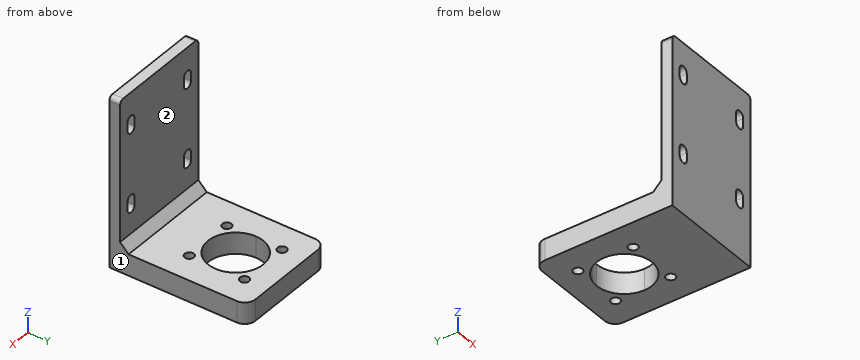
```python
from build123d import *

# Parameters (mm, degrees)
SKETCH_1_R               = 2.15
EXTRUDE_1_DEPTH          = 10
SKETCH_2_W               = 50
SKETCH_2_H               = 10
EXTRUDE_2_DEPTH          = 5
SKETCH_3_W               = 50
SKETCH_3_H               = 5
EXTRUDE_3_DEPTH          = 70
CUT_EXTRUDE_1_DEPTH      = 104.07764064
CUT_EXTRUDE_1_DEPTH_BACK = 20
FILLET_1_R               = 5
FILLET_2_R               = 2
SKETCH_9_W               = 4
SKETCH_9_H               = 4
EXTRUDE_4_DEPTH          = 4
SKETCH_13_W              = 4
SKETCH_13_H              = 4
EXTRUDE_6_DEPTH          = 46
CUT_EXTRUDE_2_DEPTH      = 101.623058987


with BuildPart() as part:
    # 草图1 → 凸台-拉伸1 (new body)
    # profile 1 of 3: a face of its own
    with BuildSketch(Plane.XY):
        with BuildLine():
            Line((13, 6), (25, 6))
            Line((25, 6), (25, 30))
            Line((25, 30), (0, 30))
            Line((0, 30), (0, 19))
            ThreePointArc((0, 19), (9.192388155, 15.192388155), (13, 6))
        make_face()
        with Locations((12, 19)):
            Circle(SKETCH_1_R, mode=Mode.SUBTRACT)
    # profile 2 of 3: a face of its own
    with BuildSketch(Plane.XY):
        with BuildLine():
            Line((-25, 19), (-25, 6))
            Line((-25, 6), (-13, 6))
            ThreePointArc((-13, 6), (-9.192388155, 15.192388155), (0, 19))
            Line((0, 19), (0, 30))
            Line((0, 30), (-25, 30))
            Line((-25, 30), (-25, 19))
        make_face()
        with Locations((-12, 19)):
            Circle(SKETCH_1_R, mode=Mode.SUBTRACT)
    # profile 3 of 3: a face of its own
    with BuildSketch(Plane.XY):
        with BuildLine():
            Line((-25, -30), (25, -30))
            Line((25, -30), (25, -27))
            Line((25, -27), (25, -7))
            Line((25, -7), (25, 6))
            Line((25, 6), (13, 6))
            ThreePointArc((13, 6), (0, -7), (-13, 6))
            Line((-13, 6), (-25, 6))
            Line((-25, 6), (-25, -30))
        make_face()
        with Locations((-12, -7)):
            Circle(SKETCH_1_R, mode=Mode.SUBTRACT)
        with Locations((12, -7)):
            Circle(SKETCH_1_R, mode=Mode.SUBTRACT)
    extrude(amount=EXTRUDE_1_DEPTH)

    # 草图2 → 凸台-拉伸2 (add)
    with BuildSketch(Plane.XZ.offset(30)):
        with Locations((0, 5)):
            Rectangle(SKETCH_2_W, SKETCH_2_H)
    extrude(amount=EXTRUDE_2_DEPTH)

    # 草图3 → 凸台-拉伸3 (add)
    with BuildSketch(Plane.XY.offset(10)):
        with Locations((0, -32.5)):
            Rectangle(SKETCH_3_W, SKETCH_3_H)
    extrude(amount=EXTRUDE_3_DEPTH)

    # 草图8 → 切除-拉伸1 (cut, two sides: drawn at the far end of the back side and taken through both)
    with BuildSketch(Plane(origin=(0, -30, 0), x_dir=(1, 0, 0), z_dir=(0, 1, 0)).offset(-CUT_EXTRUDE_1_DEPTH_BACK)):
        with BuildLine():
            Line((-20.25, -66.9), (-20.25, -63.1))
            ThreePointArc((-20.25, -63.1), (-18, -60.85), (-15.75, -63.1))
            Line((-15.75, -63.1), (-15.75, -66.9))
            ThreePointArc((-15.75, -66.9), (-18, -69.15), (-20.25, -66.9))
        make_face()
        with BuildLine():
            Line((-15.75, -26.1), (-15.75, -29.9))
            ThreePointArc((-15.75, -29.9), (-18, -32.15), (-20.25, -29.9))
            Line((-20.25, -29.9), (-20.25, -26.1))
            ThreePointArc((-20.25, -26.1), (-18, -23.85), (-15.75, -26.1))
        make_face()
        with BuildLine():
            Line((20.25, -66.9), (20.25, -63.1))
            ThreePointArc((20.25, -63.1), (18, -60.85), (15.75, -63.1))
            Line((15.75, -63.1), (15.75, -66.9))
            ThreePointArc((15.75, -66.9), (18, -69.15), (20.25, -66.9))
        make_face()
        with BuildLine():
            Line((15.75, -26.1), (15.75, -29.9))
            ThreePointArc((15.75, -29.9), (18, -32.15), (20.25, -29.9))
            Line((20.25, -29.9), (20.25, -26.1))
            ThreePointArc((20.25, -26.1), (18, -23.85), (15.75, -26.1))
        make_face()
    extrude(amount=CUT_EXTRUDE_1_DEPTH + CUT_EXTRUDE_1_DEPTH_BACK, mode=Mode.SUBTRACT)

    # 圆角1
    fillet_1_edges = [part.edges().sort_by_distance(p)[0] for p in [
        (-25, 30, 5),
        (25, 30, 5),
    ]]
    fillet(fillet_1_edges, radius=FILLET_1_R)

    # 圆角2
    fillet_2_edges = [part.edges().sort_by_distance(p)[0] for p in [
        (25, -32.5, 80),
        (-25, -32.5, 80),
    ]]
    fillet(fillet_2_edges, radius=FILLET_2_R)

    # 草图9 → 凸台-拉伸4 (add)
    with BuildSketch(Plane(origin=(0, -30, 0), x_dir=(1, 0, 0), z_dir=(0, 1, 0))):
        with Locations((23, -12)):
            Rectangle(SKETCH_9_W, SKETCH_9_H)
    extrude(amount=EXTRUDE_4_DEPTH)

    # 草图13 → 凸台-拉伸6 (add)
    with BuildSketch(Plane.ZY.offset(-21)):
        with Locations((12, -28)):
            Rectangle(SKETCH_13_W, SKETCH_13_H)
    extrude(amount=EXTRUDE_6_DEPTH)

    # 草图14 → 切除-拉伸2 (cut, through all)
    with BuildSketch(Plane(origin=(25, 0, 0), x_dir=(0, 0, -1), z_dir=(1, 0, 0))):
        Polygon((-10, -26), (-14, -30), (-14, -26), align=None)
    extrude(amount=-CUT_EXTRUDE_2_DEPTH, mode=Mode.SUBTRACT)


solid = part.part
```
The listing builds one solid part. Answer for the finished solid, in the listing's coordinates (mm). Face numbers are marked on the shaded views. A direction names the side the tool comes from. Round coordinates to 2 decimals unless told otherwise and drop trailing zeros. Write each loop counter-clockwise with the first axis right and the second up, starting at its lowest first coordinate (ties: lowest second). Pieces come first, ordered by that corner, then holes. Notation, with made-up numbers: (-40, -17.75) -> (9, -17.75) arc R22 cw to (9, -0.75) -> close; hole circle Ø11 at (87, -14.75). An arc over 180 degrees is marked (long way). Write item = value, one per line.
1) Given pin 1 (2.5 mm diameter, centred on x = 12, y = -7, fed in from +Z); pin 2 (4 mm diameter, centred on x = 9, y = -23.5, fed in from +Z); pin 3 (8 mm diameter, centred on x = 12, z = 29, fed in from +Y), each flat-ended and moving along its own axis, determine where each tip first touches the part or whether it passes through.
Check values:
pin_1 = through
pin_2 = 10
pin_3 = -30
2) Section D-D on y = -3 is taken. Write down the section's boundary in (x, z).
Check values:
outline = (-25, 0) -> (-9.38, 0) -> (-9.38, 10) -> (-25, 10) -> close; (9.38, 0) -> (25, 0) -> (25, 10) -> (9.38, 10) -> close
3) Straight lines are drawn through the part: line 1 along Y through (x, z) = (-12, 2.5); line 2 along Y through (x, z) = (20, 19); line 3 along Z through (x, y) = (14, 4). For each, find the intervals that lie inside material, in ascending order. Write a range as [from, to].
Check values:
line_1 = [-35, -9.15], [-4.85, 1], [11, 16.85], [21.15, 30]
line_2 = [-35, -30]
line_3 = [0, 10]
4) Which of the six approach directions +Z, -Z, +X, -X, +Y, -Y give full straight-line access (tool end or side, diameter ignored) to the marked faces 1 and 2?
Check values:
face_1 = +Z, -Z, +X, +Y, -Y
face_2 = +Z, +X, -X, +Y
5) Section B-B on z = 28 is taken. Write down the section's boundary in (x, y).
Check values:
outline = (-25, -35) -> (-20.25, -35) -> (-20.25, -30) -> (-25, -30) -> close; (-15.75, -35) -> (15.75, -35) -> (15.75, -30) -> (-15.75, -30) -> close; (20.25, -35) -> (25, -35) -> (25, -30) -> (20.25, -30) -> close
6) Section A-A on x = 18 is taken. Write down the section's boundary in (y, z).
Check values:
outline = (-35, 0) -> (30, 0) -> (30, 10) -> (-26, 10) -> (-30, 14) -> (-30, 23.85) -> (-35, 23.85) -> close; (-35, 32.15) -> (-30, 32.15) -> (-30, 60.85) -> (-35, 60.85) -> close; (-35, 69.15) -> (-30, 69.15) -> (-30, 80) -> (-35, 80) -> close
7) Section C-C on x = 5 is taken. Write down the section's boundary in (y, z).
Check values:
outline = (-35, 0) -> (-6, 0) -> (-6, 10) -> (-26, 10) -> (-30, 14) -> (-30, 80) -> (-35, 80) -> close; (18, 0) -> (30, 0) -> (30, 10) -> (18, 10) -> close
